Design review of the part shown in the three views and the two pictorial views. Dimensions are in mm from the part's minimum x, y and z. Coordinates: 2 decimals unless noted, no trailing zeros. Loops run counter-clockwise (first coordinate to the right, second up) from the corner with the lowest first, then second, coordinate; pieces in that order, holes last.
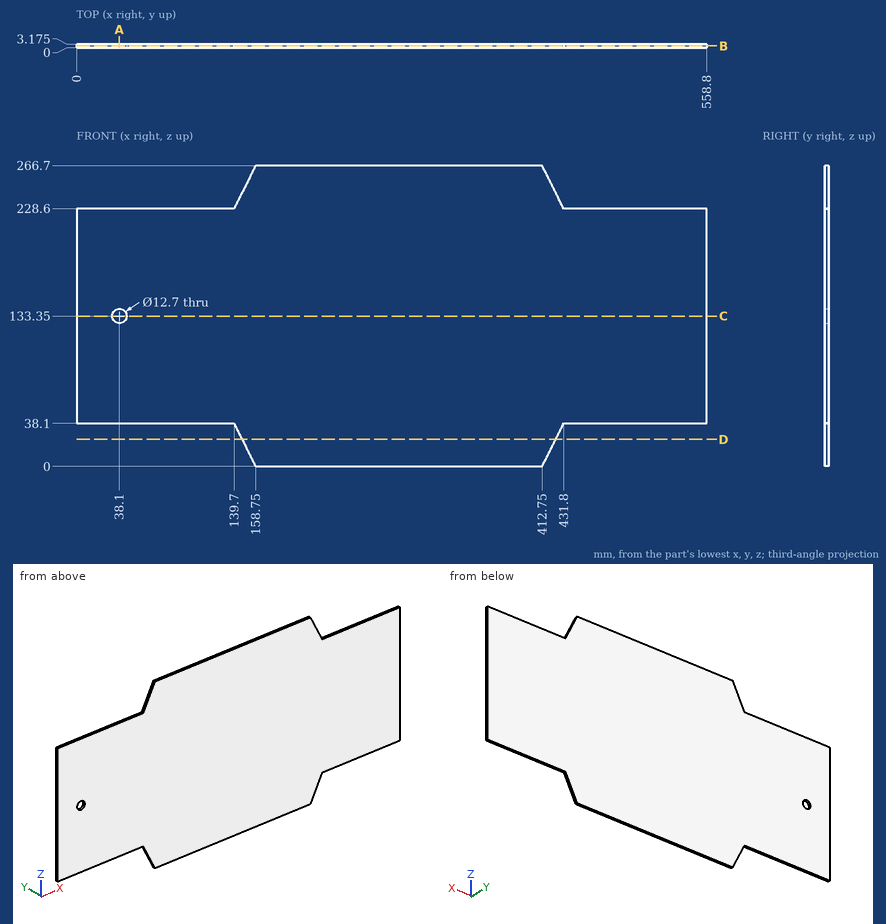
Q1. Consider section D-D (z = 24). State the section outline as (x, y) points (3 decimals).
Q2. Consider section A-A (x = 38.1). State the section outline as (y, z) points (3 decimals).
Q3. Consider section C-C (z = 133.35). State the section outline as (x, y) points (3 decimals).
Q4. Wall thickness on probe 1 along X at (y, z) = (1.7, 133.35); probe 2 along Z at (x, y) = (448.5, 2.6); probe 3 along Z at (x, y) = (38.1, 2.35): over which ranges is each line inside the solid? List them lowest first.
Q5. Consider section B-B (y = 1.45). State the section outline as (x, z) points, then the cut area to 3 significant figures.
Q6. For pin 1 Ø1.6 at (x, y) = (526, 2.5) entering from +Z; pin 2 Ø6 at (x, z) = (276.5, 111.5) entering from -Y; pin 3 Ø1.6 at (x, y) = (78, 2) entering from -Z, all flat-tipped, find the tip position at first contact; note any pin that passes through.
Model answer:
1. outline: (146.75, 0) - (424.75, 0) - (424.75, 3.175) - (146.75, 3.175) - close
2. outline: (0, 38.1) - (3.175, 38.1) - (3.175, 127) - (0, 127) - close; (0, 139.7) - (3.175, 139.7) - (3.175, 228.6) - (0, 228.6) - close
3. outline: (0, 0) - (31.75, 0) - (31.75, 3.175) - (0, 3.175) - close; (44.45, 0) - (558.8, 0) - (558.8, 3.175) - (44.45, 3.175) - close
4. probe 1: x = 0 to 31.75, 44.45 to 558.8
4. probe 2: z = 38.1 to 228.6
4. probe 3: z = 38.1 to 127, 139.7 to 228.6
5. outline: (0, 38.1) - (139.7, 38.1) - (158.75, 0) - (412.75, 0) - (431.8, 38.1) - (558.8, 38.1) - (558.8, 228.6) - (431.8, 228.6) - (412.75, 266.7) - (158.75, 266.7) - (139.7, 228.6) - (0, 228.6) - close; hole circle Ø12.7 at (38.1, 133.35)
5. area: 127,000 mm2
6. pin 1: stops at z = 228.6
6. pin 2: stops at y = 0
6. pin 3: stops at z = 38.1
